from build123d import *

# Parameters (mm, degrees)
F0_R     = 10
F0_R_2   = 2
F1_DEPTH = 6.35


# Not quite as in the source:
# - a length typed as a fraction of an inch, garbled in the dataset ("3 / 203.2 mm" for 3/8 in), is restored


with BuildPart() as f1:
    # F0 (on Front) → F1 (new body)
    with BuildSketch(Plane.XZ):
        Circle(F0_R)
        with BuildLine():
            ThreePointArc((0, 7.5), (5.3033008589, 5.3033008589), (7.5, 0))
            ThreePointArc((7.5, 0), (5.3033008589, -5.3033008589), (0, -7.5))
            ThreePointArc((0, -7.5), (-5.3033008589, -5.3033008589), (-7.5, 0))
            ThreePointArc((-7.5, 0), (-5.3033008589, 5.3033008589), (0, 7.5))
        make_face(mode=Mode.SUBTRACT)
        with BuildLine():
            ThreePointArc((0, -7.5), (5.3033008589, -5.3033008589), (7.5, 0))
            Line((7.5, 0), (3.75, 0))
            ThreePointArc((3.75, 0), (2.6516504294, -2.6516504294), (0, -3.75))
            Line((0, -3.75), (0, -7.5))
        make_face()
        with BuildLine():
            Line((0, 3.75), (0, 7.5))
            ThreePointArc((0, 7.5), (-5.3033008589, 5.3033008589), (-7.5, 0))
            Line((-7.5, 0), (-3.75, 0))
            ThreePointArc((-3.75, 0), (-2.6516504294, 2.6516504294), (0, 3.75))
        make_face()
        with BuildLine():
            ThreePointArc((0, -3.75), (2.6516504294, -2.6516504294), (3.75, 0))
            ThreePointArc((3.75, 0), (2.6516504294, 2.6516504294), (0, 3.75))
            ThreePointArc((0, 3.75), (-2.6516504294, 2.6516504294), (-3.75, 0))
            ThreePointArc((-3.75, 0), (-2.6516504294, -2.6516504294), (0, -3.75))
        make_face()
        Circle(F0_R_2, mode=Mode.SUBTRACT)
    extrude(amount=F1_DEPTH)


solid = f1.part
For this review, take the finished solid that the model builds, in its own axes (mm). A direction names the side the tool comes from. Coordinates: 2 decimals unless noted, no trailing zeros. Loops run counter-clockwise (first coordinate to the right, second up) from the corner with the lowest first, then second, coordinate; pieces in that order, holes last. Notation, with made-up numbers: (49, 68) -> (107, 68) arc R19 ccw to (107, 82) -> close; hole circle Ø7 at (14, -11.5). An arc over 180 degrees is marked (long way). Write each question's results on one line, items separated by ' | '.
Q1. Machinability: for faces 5 (the flat face through (0, -3, 6)), 6 (the flat face through (-2.4, -6.35, 0.1)), which of the approach directions +Z, -Z, +X, -X, +Y, -Y give a long, thin tool a straight path to every point of the face, cutting with its end or side? Answer none if there is none.
Taken from the geometry:
face 5: +Y, -Y | face 6: +Z, -Z, +X, -X, -Y
Q2. Add section A-A, the plane x = 7.25. State the section outline as (y, z) points.
Taken from the geometry:
outline: (-6.35, -6.89) -> (0, -6.89) -> (0, 0) -> (-6.35, 0) -> close; (-6.35, 1.92) -> (0, 1.92) -> (0, 6.89) -> (-6.35, 6.89) -> close
Q3. Mouldability with a two-part tool opening along X and no side actions: class faces 1 (the cylindrical face through (2.7, -3.1, 2.6)), 2 (the cylindrical face through (-2.17, -3.13, -9.76)), 3 (the flat face through (-2.4, 0, 0.1)), 4 (the cylindrical face through (-5.245, -3.131, -5.361)) as +X half, -X half, draft (parallel to the pull), parting line (faces both ways), or undercut.
Taken from the geometry:
face 1: undercut | face 2: parting line | face 3: draft | face 4: undercut
Q4. To check wall thickness, follow line 1 along X through (y, z) = (-4.75, -1.25); line 2 along Z through (x, y) = (-0.25, -0.25); line 3 along X through (y, z) = (-5.5, -0.75). State the ranges of each line that lie inside material, in increasing order. Write a range as [from, to].
Taken from the geometry:
line 1: [-9.92, -7.4], [-3.54, -1.56], [1.56, 9.92] | line 2: [-10, -7.5], [-3.74, -1.98], [1.98, 10] | line 3: [-9.97, -7.46], [-3.67, -1.85], [1.85, 9.97]
Q5. Add section B-B, the plane z = -1.5. State the section outline as (x, y) points, then the cut area to 3 significant figures.
Taken from the geometry:
outline: (-9.89, -6.35) -> (-7.35, -6.35) -> (-7.35, 0) -> (-9.89, 0) -> close; (-3.44, -6.35) -> (-1.32, -6.35) -> (-1.32, 0) -> (-3.44, 0) -> close; (1.32, -6.35) -> (9.89, -6.35) -> (9.89, 0) -> (1.32, 0) -> close | area: 83.9 mm²
Q6. Add section C-C, the plane y = -2.25. State the section outline as (x, z) points.
Taken from the geometry:
outline: circle Ø20 at (0, 0); hole (-7.5, 0) arc R7.5 ccw to (0, -7.5) -> (0, -3.75) arc R3.75 cw to (-3.75, 0) -> close; hole circle Ø4 at (0, 0); hole (0, 3.75) arc R3.75 cw to (3.75, 0) -> (7.5, 0) arc R7.5 ccw to (0, 7.5) -> close
Q7. Add section D-D, the plane z = 2.5. State the section outline as (x, y) points, then the cut area to 3 significant figures.
Taken from the geometry:
outline: (-9.68, -6.35) -> (2.8, -6.35) -> (2.8, 0) -> (-9.68, 0) -> close; (7.07, -6.35) -> (9.68, -6.35) -> (9.68, 0) -> (7.07, 0) -> close | area: 95.8 mm²
Q8. For pin 1 Ø1.9 at (x, y) = (-6.5, -4) entering from -Z; pin 2 Ø2 at (x, y) = (-8, -2.5) entering from -Z; pin 3 Ø1.5 at (x, y) = (1, -3) entering from +Z, all flat-tipped, find the tip position at first contact; note any pin that passes through.
Taken from the geometry:
pin 1: z = -8.32 | pin 2: z = -7.14 | pin 3: z = 10
